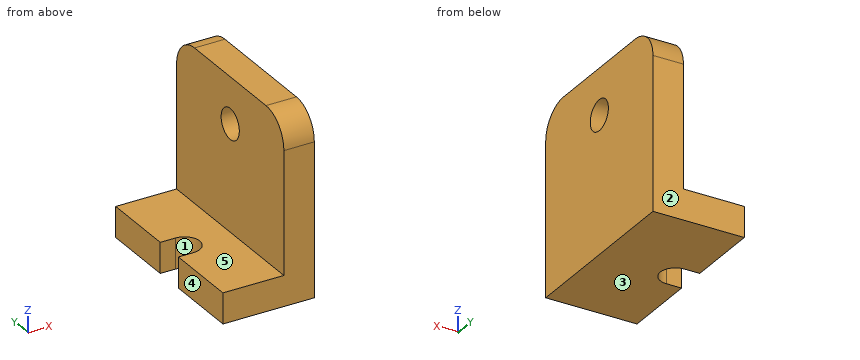
```python
from build123d import *

# Parameters (mm, degrees)
F1_DEPTH = 74.999977
F2_R     = 12.7
F3_DEPTH = 25.4
F5_DEPTH = 25.4
F6_R     = 25.000001
F7_R     = 25.000001


with BuildPart() as f1:
    # F0 (on Front) → F1 (new body, symmetric)
    with BuildSketch(Plane.XZ):
        Polygon((-76.2, 0), (0, 0), (0, 152.4), (-25.4, 152.4), (-25.4, 25.4), (-76.2, 25.4), align=None)
    extrude(amount=F1_DEPTH, both=True)

    # F2 (on Right) → F3 (cut)
    with BuildSketch(Plane.YZ):
        with Locations((0, 113.898948)):
            Circle(F2_R)
    extrude(amount=-F3_DEPTH, mode=Mode.SUBTRACT)

    # F4 (on Top) → F5 (cut)
    with BuildSketch(Plane.XY):
        with BuildLine():
            ThreePointArc((-63.519787, -12.7), (-50.819787, 0), (-63.519787, 12.7))
            Line((-63.519787, 12.7), (-76.219787, 12.7))
            Line((-76.219787, 12.7), (-76.219787, -12.7))
            Line((-76.219787, -12.7), (-63.519787, -12.7))
        make_face()
    extrude(amount=F5_DEPTH, mode=Mode.SUBTRACT)

    # F6
    f6_edges = [f1.edges().sort_by_distance(p)[0] for p in [
        (-12.7, -74.999977, 152.4),
    ]]
    fillet(f6_edges, radius=F6_R)

    # F7
    f7_edges = [f1.edges().sort_by_distance(p)[0] for p in [
        (-12.7, 74.999977, 152.4),
    ]]
    fillet(f7_edges, radius=F7_R)


solid = f1.part
```
CAD build for the part. Positions are in the model's coordinates, mm. Face numbers are marked on the shaded views. A direction names the side the tool comes from. Round coordinates to 2 decimals unless told otherwise and drop trailing zeros. Loops run counter-clockwise (first coordinate to the right, second up) from the corner with the lowest first, then second, coordinate; pieces in that order, holes last. Notation, with made-up numbers: (17, 42.25) - (32, 42.25) arc R26 ccw to (32, 66.25) - close; hole circle Ø9 at (52.25, 21.5). An arc over 180 degrees is marked (long way). Return JSON: item names as keys, results as strings. Group by question number.
Q1. Band-saw the part on D-D on x = -12. Give the cut face in (y, z), plus the area to 3 significant figures.
Q2. Tool access for the marked faces 4 and 5: list every direction of +Z, -Z, +X, -X, +Y, -Y with a clear straight run to the whole face (end or side of a thin tool).
Q3. Two-plate mould, pull along Y, no slides. Class the marked faces 1, 2 and 3: +Y half, -Y half, draft (parallel to the pull), parting line (faces both ways), or undercut.
Q4. Band-saw the part on A-A on x = -69. Give the cut face in (y, z), plus the area to 3 significant figures.
Q5. Band-saw the part on C-C on z = 12.5. Give the cut face in (x, y), plus the area to 3 significant figures.
Q6. Drill centre lines: line 1 along Z through (x, y) = (-10.75, 0); line 2 along X through (y, z) = (65, 60); line 3 along Z through (x, y) = (-39, -38). Where is each one in solid material? Low to high. Write a range as [from, to].
Q7. Band-saw the part on B-B on y = 0. Give the cut face in (x, z), plus the area to 3 significant figures.
Q8. Flat gauge pins, fed straight in: pin 1 Ø1.5 at (x, y) = (-68, -16.5) entering from +Z; pin 2 Ø2 at (y, z) = (-26.5, 45.5) entering from -X. Where does each tip first touch, or does it go through?
Solutions:
{
 "1": {"outline": "(-75, 0) - (75, 0) - (75, 127.4) arc R25 ccw to (50, 152.4) - (-50, 152.4) arc R25 ccw to (-75, 127.4) - close; hole circle Ø25.4 at (0, 113.9)", "area": "22,100 mm^2"},
 "2": {"face 4": "+Z, -Z, -X, +Y, -Y", "face 5": "+Z, -X, +Y, -Y"},
 "3": {"face 1": "undercut", "face 2": "+Y half", "face 3": "draft"},
 "4": {"outline": "(-75, 0) - (-12.7, 0) - (-12.7, 25.4) - (-75, 25.4) - close; (12.7, 0) - (75, 0) - (75, 25.4) - (12.7, 25.4) - close", "area": "3,160 mm^2"},
 "5": {"outline": "(-76.2, -75) - (0, -75) - (0, 75) - (-76.2, 75) - (-76.2, 12.7) - (-63.52, 12.7) arc R12.7 cw to (-63.52, -12.7) - (-76.2, -12.7) - close", "area": "10,900 mm^2"},
 "6": {"line 1": "z = [0, 101.2], [126.6, 152.4]", "line 2": "x = [-25.4, 0]", "line 3": "z = [0, 25.4]"},
 "7": {"outline": "(-50.82, 0) - (0, 0) - (0, 101.2) - (-25.4, 101.2) - (-25.4, 25.4) - (-50.82, 25.4) - close; (-25.4, 126.6) - (0, 126.6) - (0, 152.4) - (-25.4, 152.4) - close", "area": "3,870 mm^2"},
 "8": {"pin 1": "stops at z = 25.4", "pin 2": "stops at x = -25.4"}
}
